Source: CAD feature listing. Evaluate the final solid. Frame: model axes, mm. A direction names the side the tool comes from. Give positions to 0.01 mm unless a question says otherwise; leave off trailing zeros. Write each loop counter-clockwise with the first axis right and the second up, starting at its lowest first coordinate (ties: lowest second). Pieces come first, ordered by that corner, then holes.
```python
from build123d import *

# Parameters (mm, degrees)
SKETCH1_R           = 1.75
BOSS_EXTRUDE1_DEPTH = 4
SKETCH3_W           = 1.75
SKETCH3_H           = 8
BOSS_EXTRUDE2_DEPTH = 2
FILLET1_R           = 0.5
SKETCH4_W           = 4
SKETCH4_H           = 5
CUT_EXTRUDE1_DEPTH  = 4
FILLET2_R           = 0.75


with BuildPart() as part:
    # Sketch1 → Boss-Extrude1 (new, symmetric)
    with BuildSketch(Plane(origin=(0, 0, 0), x_dir=(1, 0, 0), z_dir=(0, 1, 0))):
        with BuildLine():
            Line((34.25, 0), (3.75, 0))
            ThreePointArc((3.75, 0), (-2.34080149, 2.929701074), (-0.827679139, -3.657519275))
            Line((-0.827679139, -3.657519275), (4, -4.75))
            Line((4, -4.75), (4, -7.239192993))
            ThreePointArc((4, -7.239192993), (4.407286712, -8.448847647), (5.463264382, -9.165826034))
            ThreePointArc((5.463264382, -9.165826034), (18.881654838, -11), (32.300045295, -9.165826034))
            ThreePointArc((32.300045295, -9.165826034), (33.210788376, -8.619339874), (33.713306247, -7.68361776))
            ThreePointArc((33.713306247, -7.68361776), (34.013295596, -6.222597745), (34.25, -4.75))
            Line((34.25, -4.75), (34.25, 0))
        make_face()
        Circle(SKETCH1_R, mode=Mode.SUBTRACT)
    extrude(amount=BOSS_EXTRUDE1_DEPTH, both=True)

    # Sketch3 → Boss-Extrude2 (add)
    with BuildSketch(Plane(origin=(0, 0, 4.75), x_dir=(-1, 0, 0), z_dir=(0, 0, -1))):
        with Locations((-35.125, 0)):
            Rectangle(SKETCH3_W, SKETCH3_H)
    extrude(amount=BOSS_EXTRUDE2_DEPTH)

    # Fillet1
    fillet1_edges = [part.edges().sort_by_distance(p)[0] for p in [
        (4, 4, 5.994596496),
        (4, -4, 5.994596496),
        (4.407286712, -4, 8.448847647),
        (18.881654838, -4, 11),
        (33.210788376, -4, 8.619339874),
        (34.013295596, -4, 6.222597745),
        (34.013295596, 4, 6.222597745),
        (33.210788376, 4, 8.619339874),
        (18.881654838, 4, 11),
        (4.407286712, 4, 8.448847647),
    ]]
    fillet(fillet1_edges, radius=FILLET1_R)

    # Sketch4 → Cut-Extrude1 (cut)
    with BuildSketch(Plane(origin=(0, 0, 0), x_dir=(-1, 0, 0), z_dir=(0, 0, -1))):
        with Locations((-30, 0)):
            Rectangle(SKETCH4_W, SKETCH4_H)
    extrude(amount=-CUT_EXTRUDE1_DEPTH, mode=Mode.SUBTRACT)

    # Fillet2
    fillet2_edges = [part.edges().sort_by_distance(p)[0] for p in [
        (34.25, 0, 2.75),
        (36, 0, 2.75),
    ]]
    fillet(fillet2_edges, radius=FILLET2_R)


solid = part.part
```
1. Cut plane D-D, the plane y = 0. Return the cut outline in (x, z).
2. Mould query, pull axis X, two halves, no side actions, for faces 4 (the flat face through (16, 4, 3)), 5 (the flat face through (4, 0, 6)), 6 (the flat face through (30, 2.5, 2)). Classes: +X half, -X half, draft (parallel to the pull), parting line (faces both ways), or undercut.
3. Cut plane B-B, the plane z = -1.25. Return the cut outline in (x, y).
4. Contact query for flat-ended pins moving along their axis: P1, Ø3, axis at x = 10.5, y = 2, coming from the -Z side; P2, Ø3, axis at y = -2, z = 1, coming from the +X side; P3, Ø1.8, axis at x = 35.5, y = -0.5, coming from the +Z side. Output: stop coordinate, or through.
5. Cut plane A-A, the plane y = -3. Return the cut outline in (x, z).
6. Access query for faces 1 (the flat face through (28, 0, 2)), 2 (the flat face through (16, -4, 3)), 3 (the flat face through (34.25, 0, 1)). Directions: +Z, -Z, +X, -X, +Y, -Y. A direction counts if a zero-diameter tool reaches every point of the face in a straight line with its end or side. Return the directions, or none.
7. Line query: L1, parallel to X at y = 2, z = 0.5; L2, parallel to Z at x = 18.5, y = 1.5; L3, parallel to Z at x = 0, y = -1. Output: solid intervals per line, ascending.
8. Cut plane C-C, the plane x = 0. Return the cut outline in (y, z).
Response values:
1. outline: (-0.83, 3.66) arc R3.75 ccw (long way) to (3.75, 0) - (28, 0) - (28, 4) - (32, 4) - (32, 0) - (34.25, 0) - (34.25, 2) arc R0.75 cw to (35, 2.75) - (35.25, 2.75) arc R0.75 ccw to (36, 3.5) - (36, 4.75) - (34.25, 4.75) arc R34.58 ccw to (33.71, 7.68) arc R2 ccw to (32.3, 9.17) arc R50 ccw to (5.46, 9.17) arc R2 ccw to (4, 7.24) - (4, 4.75) - close; hole circle Ø3.5 at (0, 0)
2. face 4: draft
2. face 5: -X half
2. face 6: undercut
3. outline: (-3.54, -4) - (-1.22, -4) - (-1.22, 4) - (-3.54, 4) - close; (1.22, -4) - (3.54, -4) - (3.54, 4) - (1.22, 4) - close
4. P1: stops at z = 0
4. P2: stops at x = 34.44
4. P3: stops at z = 4.75
5. outline: (-0.83, 3.66) arc R3.75 ccw (long way) to (3.75, 0) - (34.25, 0) - (34.25, 2) arc R0.75 cw to (35, 2.75) - (35.25, 2.75) arc R0.75 ccw to (36, 3.5) - (36, 4.75) - (34.25, 4.75) arc R34.58 ccw to (33.71, 7.68) arc R2 ccw to (32.3, 9.17) arc R50 ccw to (5.46, 9.17) arc R2 ccw to (4, 7.24) - (4, 4.75) - close; hole circle Ø3.5 at (0, 0)
6. face 1: -Z
6. face 2: +Z, -Z, +X, -X, -Y
6. face 3: -Z, +X, +Y, -Y
7. L1: x = -3.72 to -1.68, 1.68 to 28, 32 to 34.25
7. L2: z = 0 to 11
7. L3: z = -3.75 to -1.75, 1.75 to 3.84
8. outline: (-4, -3.75) - (4, -3.75) - (4, -1.75) - (-4, -1.75) - close; (-4, 1.75) - (4, 1.75) - (4, 3.84) - (-4, 3.84) - close
